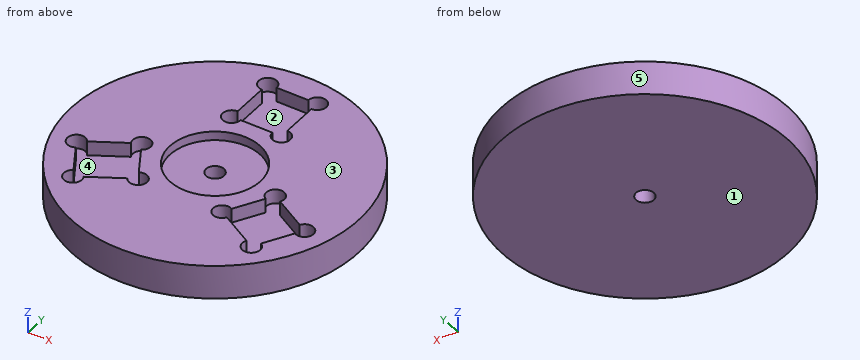
from build123d import *

# Parameters (mm, degrees)
SKETCH1_R            = 50.8
BOSS_EXTRUDE1_DEPTH  = 11.9888
SKETCH3_W            = 17.57426
SKETCH3_H            = 19.304
CUT_EXTRUDE1_DEPTH   = 5.08
SKETCH7_R            = 3.175
CORNER_RELIEFS_DEPTH = 5.08
CIRPATTERN1_COUNT    = 3
SKETCH5_R            = 16.002
MAGNET_INSET_DEPTH   = 3.175
SKETCH6_R            = 3.175
CENTRAL_HOLE_DEPTH   = 73.380681611


with BuildPart() as part:
    # Sketch1 → Boss-Extrude1 (new body)
    with BuildSketch(Plane.XY):
        with Locations(Location((0, 0, 0), (0, 0, 180))):
            Circle(SKETCH1_R)
    extrude(amount=BOSS_EXTRUDE1_DEPTH)

    # Sketch3 → Cut-Extrude1 (cut)
    with BuildSketch(Plane.XY.offset(11.9888)):
        with Locations((0, 31.877)):
            Rectangle(SKETCH3_W, SKETCH3_H)
    cut_extrude1 = extrude(amount=-CUT_EXTRUDE1_DEPTH, mode=Mode.SUBTRACT)

    # Sketch7 → corner reliefs (cut)
    with BuildSketch(Plane.XY.offset(11.9888)):
        with Locations((-8.78713, 41.529)):
            Circle(SKETCH7_R)
        with Locations((-8.78713, 22.225)):
            Circle(SKETCH7_R)
        with Locations((8.78713, 22.225)):
            Circle(SKETCH7_R)
        with Locations((8.78713, 41.529)):
            Circle(SKETCH7_R)
    corner_reliefs = extrude(amount=-CORNER_RELIEFS_DEPTH, mode=Mode.SUBTRACT)

    # CirPattern1: Cut-Extrude1, corner reliefs ×3 about axis
    cirpattern1_axis = Axis((0, 0, 0), (0, 0, 1))
    add([cut_extrude1.rotate(cirpattern1_axis, i * 360 / CIRPATTERN1_COUNT) for i in range(1, CIRPATTERN1_COUNT)], mode=Mode.SUBTRACT)
    add([corner_reliefs.rotate(cirpattern1_axis, i * 360 / CIRPATTERN1_COUNT) for i in range(1, CIRPATTERN1_COUNT)], mode=Mode.SUBTRACT)

    # Sketch5 → magnet inset (cut)
    with BuildSketch(Plane.XY.offset(11.9888)):
        Circle(SKETCH5_R)
    extrude(amount=-MAGNET_INSET_DEPTH, mode=Mode.SUBTRACT)

    # Sketch6 → central hole (cut, through all)
    with BuildSketch(Plane.XY.offset(8.8138)):
        Circle(SKETCH6_R)
    extrude(amount=-CENTRAL_HOLE_DEPTH, mode=Mode.SUBTRACT)


solid = part.part
Model file for the job. Use its own axes, mm. Face numbers are marked on the shaded views. A direction names the side the tool comes from. Give positions to 0.01 mm unless a question says otherwise; leave off trailing zeros. Order: outer loops, then holes, each group sorted by start corner. A loop starts at its lowest first (then second) coordinate and runs counter-clockwise, first axis right, second up. Notation, with made-up numbers: M 86,38 L 131,38 A29 cw 131,66 Z; hole C 44,68.25 d5. An arc over 180 degrees is marked long. Put each result on its own line as item: value. Start each with the question number.
(1) Band-saw the part on C-C on y = 23.5. Give the cut face in (x, z).
(2) Pull direction Y, two halves, no side cores. Call the marked faces 3, 4 and 5: released by +Y, released by -Y, zero draft, split by the parting line, or undercut.
(3) Band-saw the part on A-A on x = 0. Give the cut face in (y, z) (3 decimals), then the cut area to 3 significant figures.
(4) Pin check, flat tips, straight feed: pin 1 Ø4 at (x, z) = (-36, 8) entering from -Y; pin 2 Ø5.5 at (x, y) = (0, 0) entering from -Z; pin 3 Ø3 at (y, z) = (-16.5, 4.5) entering from +X; pin 4 Ø3 at (y, z) = (-34.5, 9.5) entering from -X. Stop position of each tip, or through.
(5) Band-saw the part on D-D on y = -30. Give the cut face in (x, z).
(6) Band-saw the part on B-B on z = 3. Give the cut face in (x, y) (3 decimals).
(7) Drill centre lines: L1, parallel to Y at x = 34.5, z = 9.5; L2, parallel to Y at x = 1.5, z = 11.75 (3 decimals); L3, parallel to X at y = 10.5, z = 9.75. Where is each one in solid material? Low to high. Write a range as [from, to].
(8) Tool access for the marked faces 1 and 2: list every direction of +Z, -Z, +X, -X, +Y, -Y with a clear straight run to the whole face (end or side of a thin tool).
Results below:
1. outline: M -45.04,0 L 45.04,0 L 45.04,11.99 L 11.69,11.99 L 11.69,6.91 L -11.69,6.91 L -11.69,11.99 L -45.04,11.99 Z
2. face 3: zero draft
2. face 4: undercut
2. face 5: split by the parting line
3. outline: M -50.8,0 L -3.175,0 L -3.175,8.814 L -16.002,8.814 L -16.002,11.989 L -50.8,11.989 Z; M 3.175,0 L 50.8,0 L 50.8,11.989 L 41.529,11.989 L 41.529,6.909 L 22.225,6.909 L 22.225,11.989 L 16.002,11.989 L 16.002,8.814 L 3.175,8.814 Z
3. area: 962 mm2
4. pin 1: stops at y = -37.74
4. pin 2: passes through
4. pin 3: stops at x = 48.53
4. pin 4: stops at x = -38.62
5. outline: M -41,0 L 41,0 L 41,11.99 L 34.3,11.99 L 34.3,6.91 L 28.84,6.91 L 28.84,11.99 L -28.84,11.99 L -28.84,6.91 L -34.3,6.91 L -34.3,11.99 L -41,11.99 Z
6. outline: C 0,0 d101.6; hole C 0,0 d6.35
7. L1: y = [-37.29, -29.6], [-27.15, -23.3], [-9.77, 37.29]
7. L2: y = [-50.778, -15.932], [15.932, 22.225], [41.529, 50.778]
7. L3: x = [-49.7, -12.08], [12.08, 49.7]
8. face 1: -Z, +X, -X, +Y, -Y
8. face 2: +Z
